Work out the finished part from the listing and answer in its coordinate system (mm). Face numbers are marked on the shaded views. A direction names the side the tool comes from. Give positions to 0.01 mm unless a question says otherwise; leave off trailing zeros. Order: outer loops, then holes, each group sorted by start corner. A loop starts at its lowest first (then second) coordinate and runs counter-clockwise, first axis right, second up. Notation, with made-up numbers: (1, 40.25) -> (47, 40.25) arc R22 ccw to (47, 78.25) -> close; hole circle Ø5 at (-4, 35.5). An arc over 180 degrees is marked (long way). Use a Markdown table: item, result. Add a question column.
```python
from build123d import *

# Parameters (mm, degrees)
F1_DEPTH     = 4
F2_R         = 1
F3_DEPTH     = 310
F4_T1_DEPTH  = 300
F4_T3_DEPTH  = 160
F4_T5_DEPTH  = 10
F4_T7_DEPTH  = 155
F4_T9_DEPTH  = 295
F4_T11_DEPTH = 310
F4_T17_DEPTH = 15
F4_T21_DEPTH = 160
F5_T1_DEPTH  = 300
F5_T3_DEPTH  = 160
F5_T5_DEPTH  = 10
F5_T7_DEPTH  = 155
F5_T9_DEPTH  = 295
F5_T11_DEPTH = 310
F5_T17_DEPTH = 15
F5_T21_DEPTH = 160
F6_W         = 30
F6_H         = 296
F7_DEPTH     = 2


# Not quite as in the source:
# - a fillet or chamfer that OpenCascade refuses, or shapes differently, is made with other operations: its cross-section is extruded or revolved along the edge and cut away or added


with BuildPart() as f1:
    # F0 (on Front) → F1 (new body)
    with BuildSketch(Plane.XZ):
        Polygon((251.4121359825, 250.8489221025), (-38.5878640175, 250.8489221025), (-38.5878640175, 100.8489221025), (-33.5878640175, 100.8489221025), (-33.5878640175, -49.1510778975), (251.4121359825, -49.1510778975), align=None)
    extrude(amount=F1_DEPTH)

    # F2 (on face) → F3 (cut)
    with BuildSketch(Plane.XY.offset(250.8489221025)):
        with Locations((-36.5878640175, -2)):
            Circle(F2_R)
    extrude(amount=-F3_DEPTH, mode=Mode.SUBTRACT)

    # F4: fillet of radius 2 on 6 edges, made by hand

    # F4_s2 → F4_t1 (cut)
    with BuildSketch(Plane.YZ.offset(-43.5878640175)):
        with BuildLine():
            ThreePointArc((-2, 250.8489221025), (-3.4142135624, 250.2631356648), (-4, 248.8489221025))
            Line((-4, 248.8489221025), (-4, 250.8489221025))
            Line((-4, 250.8489221025), (-2, 250.8489221025))
        make_face()
    extrude(amount=F4_T1_DEPTH, mode=Mode.SUBTRACT)

    # F4_s4 → F4_t3 (cut)
    with BuildSketch(Plane.XY.offset(95.8489221025)):
        with BuildLine():
            ThreePointArc((-36.5878640175, -4), (-38.0020775799, -3.4142135624), (-38.5878640175, -2))
            Line((-38.5878640175, -2), (-38.5878640175, -4))
            Line((-38.5878640175, -4), (-36.5878640175, -4))
        make_face()
    extrude(amount=F4_T3_DEPTH, mode=Mode.SUBTRACT)

    # F4_s6 → F4_t5 (cut)
    with BuildSketch(Plane.YZ.offset(-43.5878640175)):
        with BuildLine():
            ThreePointArc((-4, 102.8489221025), (-3.4142135624, 101.4347085401), (-2, 100.8489221025))
            Line((-2, 100.8489221025), (-4, 100.8489221025))
            Line((-4, 100.8489221025), (-4, 102.8489221025))
        make_face()
    extrude(amount=F4_T5_DEPTH, mode=Mode.SUBTRACT)

    # F4_s8 → F4_t7 (cut)
    with BuildSketch(Plane.XY.offset(-54.1510778975)):
        with BuildLine():
            ThreePointArc((-31.5878640175, -4), (-33.0020775799, -3.4142135624), (-33.5878640175, -2))
            Line((-33.5878640175, -2), (-33.5878640175, -4))
            Line((-33.5878640175, -4), (-31.5878640175, -4))
        make_face()
    extrude(amount=F4_T7_DEPTH, mode=Mode.SUBTRACT)

    # F4_s10 → F4_t9 (cut)
    with BuildSketch(Plane.YZ.offset(-38.5878640175)):
        with BuildLine():
            ThreePointArc((-4, -47.1510778975), (-3.4142135624, -48.5652914599), (-2, -49.1510778975))
            Line((-2, -49.1510778975), (-4, -49.1510778975))
            Line((-4, -49.1510778975), (-4, -47.1510778975))
        make_face()
    extrude(amount=F4_T9_DEPTH, mode=Mode.SUBTRACT)

    # F4_s12 → F4_t11 (cut)
    with BuildSketch(Plane.XY.offset(-54.1510778975)):
        with BuildLine():
            ThreePointArc((251.4121359825, -2), (250.8263495449, -3.4142135624), (249.4121359825, -4))
            Line((249.4121359825, -4), (251.4121359825, -4))
            Line((251.4121359825, -4), (251.4121359825, -2))
        make_face()
    extrude(amount=F4_T11_DEPTH, mode=Mode.SUBTRACT)


with BuildPart() as f4_tool15:
    # F4_s16 → F4_t17 (new body)
    with BuildSketch(Plane.YZ.offset(-43.5878640175)):
        with BuildLine():
            ThreePointArc((-4, 102.8489221025), (-3.4142135624, 101.4347085401), (-2, 100.8489221025))
            Line((-2, 100.8489221025), (-4, 100.8489221025))
            Line((-4, 100.8489221025), (-4, 102.8489221025))
        make_face()
    extrude(amount=F4_T17_DEPTH)

    split(bisect_by=Plane.YZ.offset(-33.5878640175), keep=Keep.TOP)


with BuildPart() as f4_tool19:
    # F4_s20 → F4_t21 (new body)
    with BuildSketch(Plane.XY.offset(105.8489221025)):
        with BuildLine():
            ThreePointArc((-31.5878640175, -4), (-33.0020775799, -3.4142135624), (-33.5878640175, -2))
            Line((-33.5878640175, -2), (-33.5878640175, -4))
            Line((-33.5878640175, -4), (-31.5878640175, -4))
        make_face()
    extrude(amount=-F4_T21_DEPTH)

    split(bisect_by=Plane.XY.offset(100.8489221025), keep=Keep.TOP)


with BuildPart() as f4_tool15_1:
    add(f4_tool15.part)

    # F4_t23: intersect F4_tool19
    add(f4_tool19.part, mode=Mode.INTERSECT)


with BuildPart() as f1_1:
    add(f1.part)

    # F4_t13: cut F4_tool15
    add(f4_tool15_1.part, mode=Mode.SUBTRACT)

    # F5: fillet of radius 2 on 6 edges, made by hand

    # F5_s2 → F5_t1 (cut)
    with BuildSketch(Plane.YZ.offset(-43.5878640175)):
        with BuildLine():
            ThreePointArc((-2, 250.8489221025), (-0.5857864376, 250.2631356648), (0, 248.8489221025))
            Line((0, 248.8489221025), (0, 250.8489221025))
            Line((0, 250.8489221025), (-2, 250.8489221025))
        make_face()
    extrude(amount=F5_T1_DEPTH, mode=Mode.SUBTRACT)

    # F5_s4 → F5_t3 (cut)
    with BuildSketch(Plane.XY.offset(95.8489221025)):
        with BuildLine():
            ThreePointArc((-36.5878640175, 0), (-38.0020775799, -0.5857864376), (-38.5878640175, -2))
            Line((-38.5878640175, -2), (-38.5878640175, 0))
            Line((-38.5878640175, 0), (-36.5878640175, 0))
        make_face()
    extrude(amount=F5_T3_DEPTH, mode=Mode.SUBTRACT)

    # F5_s6 → F5_t5 (cut)
    with BuildSketch(Plane.YZ.offset(-43.5878640175)):
        with BuildLine():
            ThreePointArc((0, 102.8489221025), (-0.5857864376, 101.4347085401), (-2, 100.8489221025))
            Line((-2, 100.8489221025), (0, 100.8489221025))
            Line((0, 100.8489221025), (0, 102.8489221025))
        make_face()
    extrude(amount=F5_T5_DEPTH, mode=Mode.SUBTRACT)

    # F5_s8 → F5_t7 (cut)
    with BuildSketch(Plane.XY.offset(-54.1510778975)):
        with BuildLine():
            ThreePointArc((-31.5878640175, 0), (-33.0020775799, -0.5857864376), (-33.5878640175, -2))
            Line((-33.5878640175, -2), (-33.5878640175, 0))
            Line((-33.5878640175, 0), (-31.5878640175, 0))
        make_face()
    extrude(amount=F5_T7_DEPTH, mode=Mode.SUBTRACT)

    # F5_s10 → F5_t9 (cut)
    with BuildSketch(Plane.YZ.offset(-38.5878640175)):
        with BuildLine():
            ThreePointArc((0, -47.1510778975), (-0.5857864376, -48.5652914599), (-2, -49.1510778975))
            Line((-2, -49.1510778975), (0, -49.1510778975))
            Line((0, -49.1510778975), (0, -47.1510778975))
        make_face()
    extrude(amount=F5_T9_DEPTH, mode=Mode.SUBTRACT)

    # F5_s12 → F5_t11 (cut)
    with BuildSketch(Plane.XY.offset(-54.1510778975)):
        with BuildLine():
            ThreePointArc((249.4121359825, 0), (250.8263495449, -0.5857864376), (251.4121359825, -2))
            Line((251.4121359825, -2), (251.4121359825, 0))
            Line((251.4121359825, 0), (249.4121359825, 0))
        make_face()
    extrude(amount=F5_T11_DEPTH, mode=Mode.SUBTRACT)


with BuildPart() as f5_tool15:
    # F5_s16 → F5_t17 (new body)
    with BuildSketch(Plane.YZ.offset(-43.5878640175)):
        with BuildLine():
            ThreePointArc((0, 102.8489221025), (-0.5857864376, 101.4347085401), (-2, 100.8489221025))
            Line((-2, 100.8489221025), (0, 100.8489221025))
            Line((0, 100.8489221025), (0, 102.8489221025))
        make_face()
    extrude(amount=F5_T17_DEPTH)

    split(bisect_by=Plane.YZ.offset(-33.5878640175), keep=Keep.TOP)


with BuildPart() as f5_tool19:
    # F5_s20 → F5_t21 (new body)
    with BuildSketch(Plane.XY.offset(105.8489221025)):
        with BuildLine():
            ThreePointArc((-31.5878640175, 0), (-33.0020775799, -0.5857864376), (-33.5878640175, -2))
            Line((-33.5878640175, -2), (-33.5878640175, 0))
            Line((-33.5878640175, 0), (-31.5878640175, 0))
        make_face()
    extrude(amount=-F5_T21_DEPTH)

    split(bisect_by=Plane.XY.offset(100.8489221025), keep=Keep.TOP)


with BuildPart() as f5_tool15_1:
    add(f5_tool15.part)

    # F5_t23: intersect F5_tool19
    add(f5_tool19.part, mode=Mode.INTERSECT)


with BuildPart() as f1_2:
    add(f1_1.part)

    # F5_t13: cut F5_tool15
    add(f5_tool15_1.part, mode=Mode.SUBTRACT)

    # F6 (on face) → F7 (join)
    with BuildSketch(Plane.XZ.offset(4)):
        with Locations((8.4121359825, 100.8489221025)):
            Rectangle(F6_W, F6_H)
    extrude(amount=F7_DEPTH)


solid = f1_2.part
```
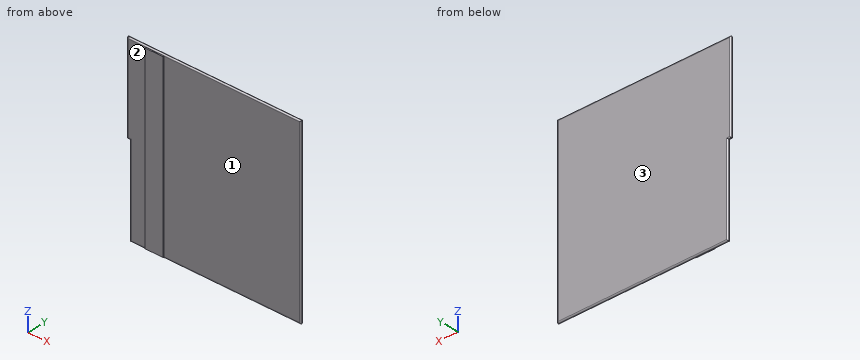
1) The part is cut by section B-B, the plane z = -5. Determine the outline of the cut face in (x, y).
2) Flat-ended cylindrical pins translate along their axes: pin 1 (3 mm diameter, centred on y = -1, z = 89.5, fed in from -X); pin 2 (1 mm diameter, centred on x = 14.5, y = -5.5, fed in from -Z); pin 3 (1 mm diameter, centred on x = 221, y = -3, fed in from -Z). Find the tip coordinate at first contact, or state that the pin passes through.
3) Straight lines are drawn through the part: line 1 (X direction, y = -1.75, z = 153.5); line 2 (Y direction, x = 102.5, z = 87); line 3 (Z direction, x = 72, y = -2.25). For each, find the intervals that lie inside material, in ascending order.
4) The part is cut by section A-A, the plane z = 109. Determine the outline of the cut face in (x, y), then the cut area to 3 significant figures.
5) The part is cut by section C-C, the plane x = 167. Determine the outline of the cut face in (y, z).
6) Which of the six approach directions +Z, -Z, +X, -X, +Y, -Y give full straight-line access (tool end or side, diameter ignored) to the marked faces 1, 2 and 3?
A:
| question | item | result |
|---|---|---|
| 1 | outline | (-31.59, -4) -> (-6.59, -4) -> (-6.59, -6) -> (23.41, -6) -> (23.41, -4) -> (249.41, -4) arc R2 ccw to (249.41, 0) -> (-31.59, 0) arc R2 ccw to start |
| 2 | pin 1 | x = -33.59 |
| 2 | pin 2 | z = -47.15 |
| 2 | pin 3 | z = -49.09 |
| 3 | line 1 | -38.57 to -37.56, -35.62 to 251.4 |
| 3 | line 2 | -4 to 0 |
| 3 | line 3 | -49.14 to 250.83 |
| 4 | outline | (-36.59, -4) -> (-6.59, -4) -> (-6.59, -6) -> (23.41, -6) -> (23.41, -4) -> (249.41, -4) arc R2 ccw to (249.41, 0) -> (-36.59, 0) arc R2 ccw to start; hole circle Ø2 at (-36.59, -2) |
| 4 | area | 1,210 mm^2 |
| 5 | outline | (-4, -47.15) arc R2 ccw to (0, -47.15) -> (0, 248.85) arc R2 ccw to (-4, 248.85) -> close |
| 6 | face 1 | +Z, -Z, +X, -Y |
| 6 | face 2 | +Z, -Z, -X, -Y |
| 6 | face 3 | +Z, -Z, +X, -X, +Y |
